Check sheet for the modelled part. Datum: model origin and axes. Units: mm. Face numbers are marked on the shaded views. A direction names the side the tool comes from. Give positions to 0.01 mm unless a question says otherwise; leave off trailing zeros. Order: outer loops, then holes, each group sorted by start corner. A loop starts at its lowest first (then second) coordinate and runs counter-clockwise, first axis right, second up. Notation, with made-up numbers: (47, 50.25) -> (66, 50.25) arc R26 cw to (66, 78.25) -> close; hole circle Ø5 at (8, 65.25). An arc over 180 degrees is marked (long way). Write each question's results on one line, items separated by ' | '.
from build123d import *

# Parameters (mm, degrees)
SKETCH_1_R               = 5
SKETCH_1_R_2             = 3.5
EXTRUDE_1_DEPTH          = 4
EXTRUDE_2_DEPTH          = 3
CUT_EXTRUDE_1_DEPTH      = 51.018502827
CUT_EXTRUDE_1_DEPTH_BACK = 51.018502827
EXTRUDE_3_DEPTH          = 1


with BuildPart() as part:
    # Sketch 1 → Extrude 1 (new, symmetric)
    with BuildSketch(Plane(origin=(0, 0, 0), x_dir=(1, 0, 0), z_dir=(0, 1, 0))):
        with Locations(Location((0, 0, 0), (0, 0, 270))):
            Circle(SKETCH_1_R)
        with Locations(Location((0, 0, 0), (0, 0, 270))):
            Circle(SKETCH_1_R_2, mode=Mode.SUBTRACT)
    extrude(amount=EXTRUDE_1_DEPTH, both=True)

    # Sketch 3 → Extrude 2 (add, symmetric)
    with BuildSketch(Plane(origin=(0, 0, 0), x_dir=(1, 0, 0), z_dir=(0, 1, 0))):
        with BuildLine():
            ThreePointArc((-4.442907632, -2.293593637), (-3.386405493, -5.288949741), (-3.182744564, -8.45863067))
            Line((-3.182744564, -8.45863067), (-5.166007589, -35.46765597))
            ThreePointArc((-5.166007589, -35.46765597), (-5.938483862, -40.935577384), (-7.435049269, -46.251137201))
            ThreePointArc((-7.435049269, -46.251137201), (0, -41.002962106), (7.435049269, -46.251137201))
            ThreePointArc((7.435049269, -46.251137201), (5.938483862, -40.935577384), (5.166007589, -35.46765597))
            Line((5.166007589, -35.46765597), (3.182744564, -8.45863067))
            ThreePointArc((3.182744564, -8.45863067), (3.386405493, -5.288949741), (4.442907632, -2.293593637))
            ThreePointArc((4.442907632, -2.293593637), (0, -5), (-4.442907632, -2.293593637))
        make_face()
        with BuildLine():
            Line((-7.890676089, -48.893638195), (7.890676089, -48.893638195))
            ThreePointArc((7.890676089, -48.893638195), (0, -41.002962106), (-7.890676089, -48.893638195))
        make_face()
    extrude(amount=EXTRUDE_2_DEPTH, both=True)

    # Sketch 4 → Cut-Extrude 1 (cut, two sides: drawn at the far end of the back side and taken through both)
    with BuildSketch(Plane(origin=(0, 3, 0), x_dir=(1, 0, 0), z_dir=(0, 1, 0)).offset(-CUT_EXTRUDE_1_DEPTH_BACK)):
        with BuildLine():
            Line((-6.517089491, -48.893638195), (6.517089491, -48.893638195))
            ThreePointArc((6.517089491, -48.893638195), (0, -42.376548704), (-6.517089491, -48.893638195))
        make_face()
    extrude(amount=CUT_EXTRUDE_1_DEPTH + CUT_EXTRUDE_1_DEPTH_BACK, mode=Mode.SUBTRACT)

    # Sketch 5 → Extrude 3 (add, symmetric)
    with BuildSketch(Plane(origin=(0, 3, 0), x_dir=(1, 0, 0), z_dir=(0, 1, 0))):
        with BuildLine():
            Line((-6.517089491, -48.893638195), (-7.890676089, -48.893638195))
            ThreePointArc((-7.890676089, -48.893638195), (0, -41.002962106), (7.890676089, -48.893638195))
            Line((7.890676089, -48.893638195), (6.517089491, -48.893638195))
            ThreePointArc((6.517089491, -48.893638195), (0, -42.376548704), (-6.517089491, -48.893638195))
        make_face()
    extrude(amount=EXTRUDE_3_DEPTH, both=True)


solid = part.part
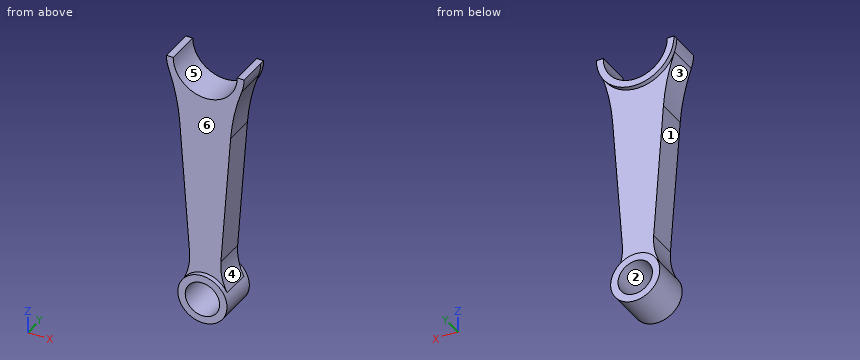
1. Access from +Z, -Z, +X, -X, +Y, -Y to the whole of each face (thin tool, end or side, straight path). Record for the marked faces 1 and 2.
Verdict:
face 1: -X, +Y, -Y | face 2: +Y, -Y
2. Section check B-B on x = 0. Record the cut outline in (y, z).
Verdict:
outline: (-4, -5) -> (4, -5) -> (4, -3.5) -> (-4, -3.5) -> close; (-4, 3.5) -> (4, 3.5) -> (4, 5) -> (3, 5) -> (3, 41) -> (4, 41) -> (4, 42.38) -> (-3, 42.38) -> (-3, 5) -> (-4, 5) -> close
3. Gauge pin test, flat ends, axial feed: pin 1 Ø6 at (x, z) = (-4, 40.5) entering from -Y; pin 2 Ø1.5 at (y, z) = (-3, 39.5) entering from +X; pin 3 Ø4 at (y, z) = (-1.5, 10.5) entering from +X; pin 4 Ø8 at (x, z) = (0, 0) entering from -Y. Record the tip position at first contact, or that the pin passes through.
Verdict:
pin 1: stops at y = -3 | pin 2: stops at x = 5.8 | pin 3: stops at x = 3.48 | pin 4: stops at y = -4
4. Material ranges on probe 1 along X at (y, z) = (-1.25, 0); probe 2 along Z at (x, y) = (1, 3.75); probe 3 along Z at (x, y) = (-1.75, 3.5), recorded low to high. Write a range as from..to.
Verdict:
probe 1: x = -5..-3.5, 3.5..5 | probe 2: z = -4.9..-3.35, 3.35..4.9, 41.07..42.45 | probe 3: z = -4.68..-3.03, 3.03..4.68, 41.2..42.62
5. Section check D-D on z = 24. Record the cut outline in (x, y), then the cut area to 3 significant figures.
Verdict:
outline: (-4.32, -3) -> (4.32, -3) -> (4.32, 3) -> (-4.32, 3) -> close | area: 51.9 mm^2
6. Section check A-A on y = 0.25. Record the cut outline in (x, z), then the cut area to 3 significant figures.
Verdict:
outline: (-7.89, 48.89) arc R7.89 ccw to (-7.44, 46.25) arc R41.21 cw to (-5.17, 35.47) -> (-3.18, 8.46) arc R11.59 cw to (-4.44, 2.29) arc R5 ccw (long way) to (4.44, 2.29) arc R11.59 cw to (3.18, 8.46) -> (5.17, 35.47) arc R41.21 cw to (7.44, 46.25) arc R7.89 ccw to (7.89, 48.89) -> (6.52, 48.89) arc R6.52 cw to (-6.52, 48.89) -> close; hole circle Ø7 at (0, 0) | area: 396 mm^2
7. Mould release check, pull along Z, two halves, no side actions. Record for the marked faces 3, 4, 5 and 6: +Z half, -Z half, draft (parallel to the pull), parting line (faces both ways), or undercut.
Verdict:
face 3: -Z half | face 4: undercut | face 5: +Z half | face 6: draft
8. Section check C-C on z = 0. Record the cut outline in (x, y).
Verdict:
outline: (-5, -4) -> (-3.5, -4) -> (-3.5, 4) -> (-5, 4) -> close; (3.5, -4) -> (5, -4) -> (5, 4) -> (3.5, 4) -> close
